Geometry: see drawing. Coordinates: mm, zero at the bounding-box minimum. A direction names the side the tool comes from. Round coordinates to 2 decimals unless told otherwise and drop trailing zeros. Loops run counter-clockwise (first coordinate to the right, second up) from the corner with the lowest first, then second, coordinate; pieces in that order, holes last. Notation, with made-up numbers: (17, 57) - (51, 57) arc R22 ccw to (51, 72) - close; hole circle Ø1 at (-36, -11). An arc over 180 degrees is marked (long way). Write item = value, one per line. Start each with the question number.
Item 1: Line query: line 1 (Y direction, x = 5.25, z = 4.75); line 2 (X direction, y = 2.75, z = 2); line 3 (Y direction, x = 14.75, z = 2.5). Output: solid intervals per line, ascending. Write a range as from..to.
Item 2: Section D-D (x = 37.5). Return loops of the section in (y, z).
Item 3: Section B-B (y = 2.9). Return loops of the section in (x, z).
Item 4: Access query for the marked faces 5 and 6. Directions: +Z, -Z, +X, -X, +Y, -Y. A direction counts if a zero-diameter tool reaches every point of the face in a straight line with its end or side. Return the directions, or none.
Item 5: Draft query along Y for the marked faces 1, 2, 3 and 4. Return one class per face: pulls with the +Y half, pulls with the -Y half, needs draft (parallel to the pull), parting line crosses it, or undercut.
Item 6: First-contact query: pin 1 (1.9 mm diameter, centred on x = 39, z = 2, fed in from -Y); pin 2 (1.9 mm diameter, centred on y = 5, z = 4.5, fed in from +X). Flat tips, straight axial feed; report the tip coordinate or a pass-through.
Item 7: Section A-A (x = 5.25). Return loops of the section in (y, z).
Item 8: Section C-C (z = 2). Return loops of the section in (x, y), plus the area to 3 significant figures.
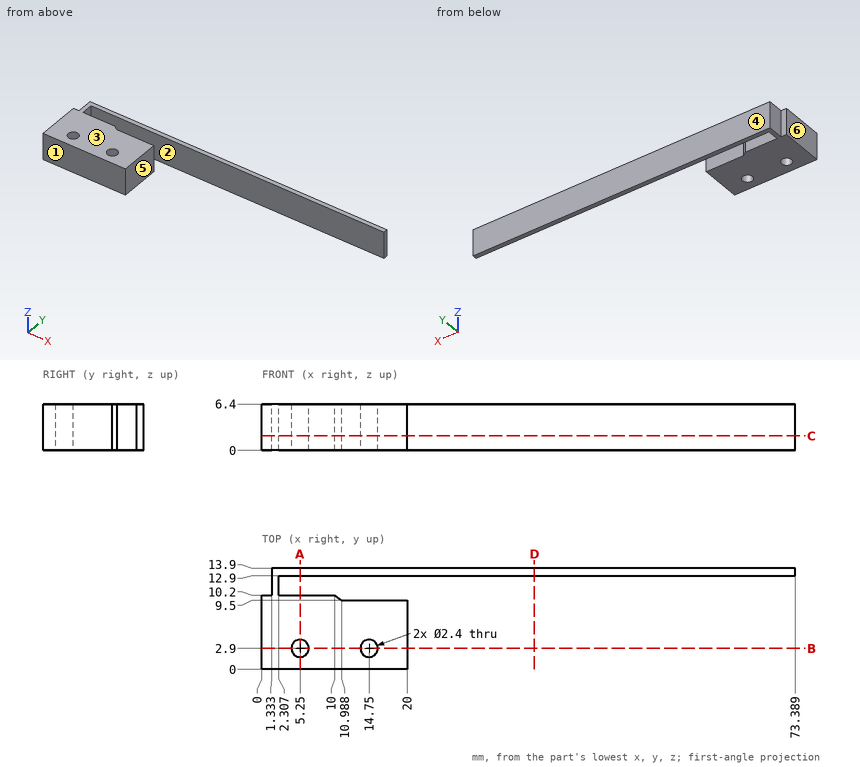
Taken from the geometry:
q1.line_1 = 0..1.7, 4.1..10.2, 12.9..13.9
q1.line_2 = 0..4.06, 6.44..13.56, 15.94..20
q1.line_3 = 0..1.7, 4.1..9.5, 12.9..13.9
q2.outline = (12.9, 0) - (13.9, 0) - (13.9, 6.4) - (12.9, 6.4) - close
q3.outline = (0, 0) - (4.05, 0) - (4.05, 6.4) - (0, 6.4) - close; (6.45, 0) - (13.55, 0) - (13.55, 6.4) - (6.45, 6.4) - close; (15.95, 0) - (20, 0) - (20, 6.4) - (15.95, 6.4) - close
q4.face_5 = +Z, -Z, +X, -Y
q4.face_6 = +Z, -Z, -X, +Y, -Y
q5.face_1 = pulls with the -Y half
q5.face_2 = undercut
q5.face_3 = needs draft
q5.face_4 = pulls with the +Y half
q6.pin_1 = 12.9
q6.pin_2 = 20
q7.outline = (0, 0) - (1.7, 0) - (1.7, 6.4) - (0, 6.4) - close; (4.1, 0) - (10.2, 0) - (10.2, 6.4) - (4.1, 6.4) - close; (12.9, 0) - (13.9, 0) - (13.9, 6.4) - (12.9, 6.4) - close
q8.outline = (0, 0) - (20, 0) - (20, 9.5) - (10.99, 9.5) - (10, 10.2) - (2.31, 10.2) - (2.31, 12.9) - (73.39, 12.9) - (73.39, 13.9) - (1.33, 13.9) - (1.33, 10.2) - (0, 10.2) - close; hole circle Ø2.4 at (5.25, 2.9); hole circle Ø2.4 at (14.75, 2.9)
q8.area = 263 mm^2
